Autodesk Inventor part; units mm, degrees
ref_plane "Work Plane1" through (3.175, 0, 0) normal (0, 0.5, 0.866) x (1, 0, 0)
ref_plane "YZ Plane" through (0, 0, 0) normal (1, 0, 0) x (0, 1, 0)
ref_plane "XZ Plane" through (0, 0, 0) normal (0, 1, 0) x (-1, 0, 0)
sketch "Sketch1" plane through (0, 0, 0) normal (0, 0, 1) x (1, 0, 0)
  line L0 (0, 0) -> (2.1167, 0)
  line L1 (6.35, 1.8331) -> (6.35, 3.175)
  line L2 (6.35, 3.175) -> (0, 3.175)
  line L3 (6.35, 1.8331) -> (3.175, 1.8331)
  line L4 (3.175, 1.8331) -> (2.1167, 0)
  line L5 (0, -0.635) -> (0, 3.81)
  line L6 (0, 3.175) -> (0, 0)
  dimension "d0" = 3.175
  dimension "d1" = 60
  dimension "d2" = 6.35
  dimension "d3" = 3.6662
  dimension "d5" = 6.35
revolve "Body" add sketch "Sketch1" angle 360 about axis through (0, 0, 0) along (1, 0, 0)
chamfer "Chamfer1" distance 0.7791 angle 45 1 edges at (6.35, -3.175, 0) measured on face at (6.35, 2.6792, -0.3995)
sketch "Sketch2" plane through (6.35, 0, 0) normal (1, 0, 0) x (0, 0, -1)
  circle A0 centre (0, 0) radius 1.8331
  line L0 (-0.9165, 1.5875) -> (0.9165, 1.5875)
  line L1 (0.9165, 1.5875) -> (1.8331, 0)
  line L2 (1.8331, 0) -> (0.9165, -1.5875)
  line L3 (0.9165, -1.5875) -> (-0.9165, -1.5875)
  line L4 (-0.9165, -1.5875) -> (-1.8331, 0)
  line L5 (-1.8331, 0) -> (-0.9165, 1.5875)
extrude "Slot" add sketch "Sketch2" against normal up to next contours L1 A0 | A0 L2 | L0 A0 | A0 L3 | L5 A0 | A0 L4
thread "Thread"
chamfer "Chamfer2" distance 0.7791 angle 45 1 edges at (0, -3.175, 0) measured on face at (3.714, 3.1339, -0.5093)
ref_plane "Work Plane1" through (3.175, 0, 0) normal (0, 0.5, 0.866) x (1, 0, 0)
equation "\"d0\" = INTI"
equation "\"d2\" = NND"
equation "\"d3\" = 1.1547 * SW"
equation "\"d5\" = NLG"
equation "\"d7\" = -0.5 * GD1 + 0.5 * NND"
equation "\"d8\" = FAWI"
equation "\"d29\" = -0.5 * GD1 + 0.5 * NND"
equation "\"d11\" = NLG"
equation "\"d13\" = -0.5 * GD1 + 0.5 * NND"
equation "\"d14\" = FAWI"
equation "\"d30\" = -0.5 * GD1 + 0.5 * NND"
equation "\"NND\" = 6.35"
equation "\"NLG\" = 6.35"
equation "\"INTI\" = 3.175"
equation "\"FAWI\" = 45deg"
equation "\"SW\" = 3.175"
equation "\"GD1\" = 4.79188"
equation "\"FAWI1\" = 44.999991deg"
equation "\"SPD\" = 3.3528"
equation "\"SEWI\" = 90deg"
equation "\"TOA\" = 30deg"
equation "\"ZLG\" = 1.7018"
equation "\"ZD\" = 3.9624"
equation "\"HHPTC\" = 1.27"
equation "\"THREADDIA\" = 6.35"
equation "\"OPR\" = 4.7752"
equation "\"E0\" = 1.155 * SW"
properties part number "ANSI B18.3 - 1/4-20 UNC x 0.25" material "Steel, Alloy"
Could you check a few things on this model? Use its own coordinates, in mm. A direction names the side the tool comes from. Round coordinates to 2 decimals unless told otherwise and drop trailing zeros. Loops run counter-clockwise (first coordinate to the right, second up) from the corner with the lowest first, then second, coordinate; pieces in that order, holes last. Notation, with made-up numbers: (30, 86) - (49, 86) arc R28 cw to (49, 113) - close; hole circle Ø6 at (5, -22.75). An arc over 180 degrees is marked (long way). Answer in a Markdown table with one row per item. Add a question column.
(1) If we section it at B-B (x = 6.25): Please give me the cut outline in (y, z).
(2) I need wall thicknesses on line 1 along Z through (x, y) = (4.75, -0.75); line 2 along Y through (x, z) = (4.75, 0.5); line 3 along Y through (x, z) = (5.75, -0.75). Which ranges of each line are inside material? Lowest first, please.
(3) For faces 1 (the face through (4.71, -0.8, 1.37)), 2 (the face through (6.35, -1, -2)), which set-ups out of +Z, -Z, +X, -X, +Y, -Y let a thin tool reach every point of the face, with its end or its side?
(4) I'm going to push flat-ended pins straight in: pin 1 (1 mm diameter, centred on x = 4, z = 1, fed in from +Y); pin 2 (2 mm diameter, centred on x = 3, y = -2.5, fed in from +Z); pin 3 (1 mm diameter, centred on x = 5.5, z = -2.5, fed in from +Y); pin 4 (2 mm diameter, centred on x = 5.5, z = 0.5, fed in from +Y) (3 decimals). Where does each tip first touch, or does it pass through?
(5) If we mould it in two halves opening along Z, with no side actions, what happens to faces 3 (the face through (3.14, -0.69, 3.1)), 4 (the face through (0, 0, 0)), 5 (the face through (2.18, -0.02, -0.11)), 6 (the face through (4.715, 0.783, 1.381))? For each: pulls with the +Z half, pulls with the -Z half, needs draft (parallel to the pull), parting line crosses it, or undercut.
Model answer:
| question | item | result |
|---|---|---|
| 1 | outline | circle Ø4.99 at (0, 0); hole (-1.59, -0.92) - (0, -1.83) - (1.59, -0.92) - (1.59, 0.92) - (0, 1.83) - (-1.59, 0.92) - close |
| 2 | line 1 | z = -3.09 to -1.4, 1.4 to 3.09 |
| 2 | line 2 | y = -3.14 to -1.59, 1.59 to 3.14 |
| 2 | line 3 | y = -2.9 to -1.59, 1.59 to 2.9 |
| 3 | face 1 | +X |
| 3 | face 2 | +Z, -Z, +X, +Y, -Y |
| 4 | pin 1 | stops at y = 3.14 |
| 4 | pin 2 | stops at z = 2.8 |
| 4 | pin 3 | stops at y = 2.47 |
| 4 | pin 4 | stops at y = 3.175 |
| 5 | face 3 | parting line crosses it |
| 5 | face 4 | needs draft |
| 5 | face 5 | undercut |
| 5 | face 6 | undercut |
